Geometry check sheet. Reference: the model listing, model coordinates, mm. Give positions to 0.01 mm unless a question says otherwise; leave off trailing zeros. Order: outer loops, then holes, each group sorted by start corner. A loop starts at its lowest first (then second) coordinate and runs counter-clockwise, first axis right, second up. Notation, with made-up numbers: M 1,58.25 L 44,58.25 A19 cw 44,69.25 Z; hole C 15.5,77 d5. An arc over 180 degrees is marked long. Answer as a JSON object with one key per item and string values. Group by question number.
from build123d import *

# Parameters (mm, degrees)
SKETCH_3_R      = 3
SKETCH_3_R_2    = 2
SKETCH_3_R_3    = 1.5
SKETCH_3_R_4    = 5
EXTRUDE_1_DEPTH = 2


with BuildPart() as part:
    # 草图3 → 凸台-拉伸1 (new body)
    with BuildSketch(Plane.XY):
        with BuildLine():
            Line((-46.5, 63), (-37.576612526, 61.656694359))
            ThreePointArc((-37.576612526, 61.656694359), (-11.38853896, 19.746708007), (34.06116735, 39.152540881))
            Line((34.06116735, 39.152540881), (41, 39.152540881))
            Line((41, 39.152540881), (45, 31.317051182))
            Line((45, 31.317051182), (45, 25.109783315))
            Line((45, 25.109783315), (15, -39.82))
            ThreePointArc((15, -39.82), (0, -54.82), (-15, -39.82))
            Line((-15, -39.82), (-45, 25.109783315))
            add(Edge.make_bspline(
                [(-45, 25.109783315), (-46.274240542, 26.725120767), (-46.5, 28.773494756)],
                knots=[0, 0, 0, 1, 1, 1], degree=2))
            Line((-46.5, 28.773494756), (-46.5, 63))
        make_face()
        with Locations((0, -1.82)):
            Circle(SKETCH_3_R, mode=Mode.SUBTRACT)
        with Locations((0, 13.5)):
            Circle(SKETCH_3_R_2, mode=Mode.SUBTRACT)
        with Locations((-30.0520382, 25.9479618)):
            Circle(SKETCH_3_R_2, mode=Mode.SUBTRACT)
        with Locations((-42.5, 56)):
            Circle(SKETCH_3_R_2, mode=Mode.SUBTRACT)
        with Locations((30.0520382, 25.9479618)):
            Circle(SKETCH_3_R_2, mode=Mode.SUBTRACT)
        with Locations((0, -20.82)):
            Circle(SKETCH_3_R, mode=Mode.SUBTRACT)
        with Locations((0, -39.82)):
            Circle(SKETCH_3_R, mode=Mode.SUBTRACT)
        with Locations((-25, -1.990216685)):
            Circle(SKETCH_3_R_3, mode=Mode.SUBTRACT)
        with Locations((-25, 13.509783315)):
            Circle(SKETCH_3_R_3, mode=Mode.SUBTRACT)
        with Locations(Location((25, 13.509783315, 0), (0, 0, 180))):
            Circle(SKETCH_3_R_3, mode=Mode.SUBTRACT)
        with Locations(Location((25, -1.990216685, 0), (0, 0, 180))):
            Circle(SKETCH_3_R_3, mode=Mode.SUBTRACT)
        with Locations((-12.5, -11.405108343)):
            Circle(SKETCH_3_R_4, mode=Mode.SUBTRACT)
        with Locations((-12.5, 5.844891657)):
            Circle(SKETCH_3_R_4, mode=Mode.SUBTRACT)
        with Locations(Location((12.5, 5.844891657, 0), (0, 0, 180))):
            Circle(SKETCH_3_R_4, mode=Mode.SUBTRACT)
        with Locations(Location((12.5, -11.405108343, 0), (0, 0, 180))):
            Circle(SKETCH_3_R_4, mode=Mode.SUBTRACT)
    extrude(amount=EXTRUDE_1_DEPTH)


solid = part.part
1. Cross-section at C-C (x = -25). Record the cut outline in (y, z).
2. Depth check by flat-ended pin: pin 1 (2.5 mm diameter, centred on x = 25, y = -1.99, fed in from -Z) (1 decimal). Enter the tip coordinate at first touch or a pass-through.
3. Cross-section at A-A (x = -42.5). Record the cut outline in (y, z), and give its area (3 significant figures).
4. Cross-section at D-D (z = 0.75). State how many separate pieces and enclosed holes the cut face has, and give its area (3 significant figures).
5. Cross-section at B-B (y = -20.82). Record the cut outline in (x, z), and give its area (3 significant figures).
6. Release check for a two-part mould opening along X. For faces 1 (the flat face through (30.21, -6.9, 0.99)), 2 (the cylindrical face through (26.5, -2.06, 0.99)), 3 (the flat face through (0, 5, 0)) record: released by +X, released by -X, zero draft, split by the parting line, or undercut.
7. Thickness scan on line 1 along Y through (x, z) = (0, 1.45); line 2 along Y through (x, z) = (25, 1.1); line 3 along X through (y, z) = (-12.5, 0.55). Record the ranges inside material, lowest first. Write a range as [from, to].
Report:
{
 "1": {"outline": "M -18.18,0 L -3.49,0 L -3.49,2 L -18.18,2 Z; M -0.49,0 L 12.01,0 L 12.01,2 L -0.49,2 Z; M 15.01,0 L 27.38,0 L 27.38,2 L 15.01,2 Z"},
 "2": {"pin 1": "passes through"},
 "3": {"outline": "M 19.7,0 L 54,0 L 54,2 L 19.7,2 Z; M 58,0 L 62.4,0 L 62.4,2 L 58,2 Z", "area": "77.4 mm2"},
 "4": {"separate pieces": "1", "enclosed holes": "15", "area": "4,230 mm2"},
 "5": {"outline": "M -23.78,0 L -3,0 L -3,2 L -23.78,2 Z; M 3,0 L 23.78,0 L 23.78,2 L 3,2 Z", "area": "83.1 mm2"},
 "6": {"face 1": "released by +X", "face 2": "undercut", "face 3": "zero draft"},
 "7": {"line 1": "y = [-54.82, -42.82], [-36.82, -23.82], [-17.82, -4.82], [1.18, 11.5], [15.5, 18]", "line 2": "y = [-18.18, -3.49], [-0.49, 12.01], [15.01, 27.38]", "line 3": "x = [-27.62, -17.38], [-7.62, 7.62], [17.38, 27.62]"}
}
